Autodesk Inventor part; units mm, degrees
ref_plane "YZ Plane" through (0, 0, 0) normal (1, 0, 0) x (0, 1, 0)
ref_plane "XZ Plane" through (0, 0, 0) normal (0, 1, 0) x (-1, 0, 0)
ref_plane "XY Plane" through (0, 0, 0) normal (0, 0, 1) x (1, 0, 0)
sketch "Sketch1" plane through (0, 0, 0) normal (0, 1, 0) x (-1, 0, 0)
  line L0 (51.8, 25) -> (-51.8, 25)
  line L1 (-51.8, 25) -> (-51.8, -25)
  line L2 (-51.8, -25) -> (51.8, -25)
  line L3 (51.8, -25) -> (51.8, 25)
  line L4 (51.8, 25) -> (-51.8, -25) construction
  line L5 (-51.8, 25) -> (51.8, -25) construction
  point P0 (0, 0)
  dimension "d0" = 103.6
  dimension "d1" = 50
extrude "Extrusion1" add sketch "Sketch1" along normal blind 3.125
sketch "Sketch2" plane through (0, 3.125, 0) normal (0, 1, 0) x (1, 0, 0)
  circle A0 centre (-32.0787, 0) radius 5.5
  point P0 (0, 0)
  dimension "d4" = 11
extrude "Extrusion2" cut sketch "Sketch2" against normal blind 3.125
sketch "Sketch3" plane through (0, 3.125, 0) normal (0, 1, 0) x (1, 0, 0)
  line L0 (34.4414, -6.7) -> (42.9414, -6.7)
  line L1 (42.9414, -6.7) -> (42.9414, 6.7)
  line L2 (42.9414, 6.7) -> (34.4414, 6.7)
  line L3 (34.4414, 6.7) -> (34.4414, -6.7)
  line L4 (34.4414, -6.7) -> (42.9414, 6.7) construction
  line L5 (42.9414, -6.7) -> (34.4414, 6.7) construction
  point P0 (0, 0)
  point P1 (38.6914, 0)
  dimension "d7" = 8.5
  dimension "d8" = 13.4
extrude "Extrusion3" cut sketch "Sketch3" against normal blind 3.125
properties part number "PARED"
Geometry check sheet. Reference: the model listing, model coordinates, mm. A direction names the side the tool comes from. Coordinates: 2 decimals unless noted, no trailing zeros. Order: outer loops, then holes, each group sorted by start corner. A loop starts at its lowest first (then second) coordinate and runs counter-clockwise, first axis right, second up. Notation, with made-up numbers: (-28, 47) - (-6, 47) arc R19 ccw to (-6, 56) - close; hole circle Ø2 at (74.5, 5.25). An arc over 180 degrees is marked (long way). One line per item, written item: value.
(1) Sectioned sample at A-A (z = 0). Enter the section's corners in (x, y) (3 decimals), and give its area (3 significant figures).
Data:
outline: (-51.8, 0) - (-37.579, 0) - (-37.579, 3.125) - (-51.8, 3.125) - close; (-26.579, 0) - (34.441, 0) - (34.441, 3.125) - (-26.579, 3.125) - close; (42.941, 0) - (51.8, 0) - (51.8, 3.125) - (42.941, 3.125) - close
area: 263 mm^2
(2) Sectioned sample at C-C (y = 2.3). Enter the section's corners in (x, z).
Data:
outline: (-51.8, -25) - (51.8, -25) - (51.8, 25) - (-51.8, 25) - close; hole circle Ø11 at (-32.08, 0); hole (34.44, -6.7) - (42.94, -6.7) - (42.94, 6.7) - (34.44, 6.7) - close
(3) Release check for a two-part mould opening along Z. For faces 3 (the face through (-51.8, 2, 0)), 4 (the face through (34.441, 2, 0)), 5 (the face through (1, 2, -25)) record: +Z half, -Z half, draft (parallel to the pull), parting line (faces both ways), or undercut.
Data:
face 3: draft
face 4: undercut
face 5: -Z half
(4) Sectioned sample at B-B (x = -36.5). Enter the section's corners in (y, z) (3 decimals).
Data:
outline: (0, -25) - (3.125, -25) - (3.125, -3.271) - (0, -3.271) - close; (0, 3.271) - (3.125, 3.271) - (3.125, 25) - (0, 25) - close
(5) Thickness scan on probe 1 along X at (y, z) = (1.6, 0); probe 2 along Z at (x, y) = (35, 1.2); probe 3 along X at (y, z) = (0.7, 1.5). Record the ranges inside material, lowest first. Write a range as from..to.
Data:
probe 1: x = -51.8..-37.58, -26.58..34.44, 42.94..51.8
probe 2: z = -25..-6.7, 6.7..25
probe 3: x = -51.8..-37.37, -26.79..34.44, 42.94..51.8
(6) Depth check by flat-ended pin: pin 1 Ø1.5 at (x, z) = (26.5, -15) entering from -Y; pin 2 Ø6.5 at (x, z) = (-32.08, 0) entering from +Y. Enter the tip coordinate at first touch or a pass-through.
Data:
pin 1: stops at y = 0
pin 2: passes through
(7) Access from +Z, -Z, +X, -X, +Y, -Y to the whole of each face (thin tool, end or side, straight path). Record for faces 1 (the face through (51.8, 2, 0)), 2 (the face through (39, 2, 6.7)).
Data:
face 1: +Z, -Z, +X, +Y, -Y
face 2: +Y, -Y
